CAD build for the part. Positions are in the model's coordinates, mm. A direction names the side the tool comes from. Coordinates: 2 decimals unless noted, no trailing zeros. Loops run counter-clockwise (first coordinate to the right, second up) from the corner with the lowest first, then second, coordinate; pieces in that order, holes last.
1) Pin check, flat tips, straight feed: pin 1 Ø2.5 at (x, z) = (22, 9) entering from +Y; pin 2 Ø10 at (x, y) = (-1.5, -20) entering from +Z; pin 3 Ø2.5 at (x, z) = (21.5, 9) entering from -Y; pin 4 Ø2.5 at (x, y) = (18, 45) entering from -Z. Stop position of each tip, or through.
2) Saw through at C-C, the plane z = 4.5. Write the cut outline in (x, y), and give its area (3 significant figures).
3) Which spindle directions (+Z, -Z, +X, -X, +Y, -Y) get a long thin tool onto all of the face, cutting with end or side? Do faces 1 (the flat face through (0, -25, 1)), 2 (the flat face through (-22, -19.15, 9)), 3 (the flat face through (0, 45, 1)), 4 (the flat face through (-20, 10, 9)). Say none if no direction does.
4) Wall check: line 1 along Y through (x, z) = (-18, 1.65); line 2 along X through (y, z) = (18.5, 8); line 3 along Z through (x, y) = (-11.5, 36). Give the ranges that are in metal, low to high.
5) Saw through at D-D, the plane x = -17.5. Write the cut outline in (y, z), and give its area (3 significant figures).
6) Saw through at B-B, the plane y = 18.5. Write the cut outline in (x, z), and give its area (3 significant figures).
7) Saw through at A-A, the plane x = 18. Write the cut outline in (y, z).
```python
from build123d import *

# Parameters (mm, degrees)
SKETCH1_W           = 40
SKETCH1_H           = 58.3
SKETCH1_R           = 1.55
SKETCH1_W_2         = 3
BOSS_EXTRUDE2_DEPTH = 2.5
SKETCH1_4_W         = 3
SKETCH1_4_H         = 58.3
BOSS_EXTRUDE3_DEPTH = 16
FILLET1_R           = 2
FILLET2_R           = 3


with BuildPart() as part:
    # Sketch1 → Boss-Extrude2 (new body)
    # profile 1 of 5: a face of its own
    with BuildSketch(Plane.XY):
        with Locations((0, 10)):
            Rectangle(SKETCH1_W, SKETCH1_H)
    # profile 2 of 5: a face of its own
    with BuildSketch(Plane.XY):
        Polygon((-23, 39.15), (-20, 39.15), (20, 39.15), (23, 39.15), (23, 50), (13, 50), (13, 45), (-13, 45), (-13, 50), (-23, 50), align=None)
        with Locations((-18, 45)):
            Circle(SKETCH1_R, mode=Mode.SUBTRACT)
        with Locations((18, 45)):
            Circle(SKETCH1_R, mode=Mode.SUBTRACT)
    # profile 3 of 5: a face of its own
    with BuildSketch(Plane.XY):
        with Locations((21.5, 10)):
            Rectangle(SKETCH1_W_2, SKETCH1_H)
    # profile 4 of 5: a face of its own
    with BuildSketch(Plane.XY):
        Polygon((20, -19.15), (-20, -19.15), (-23, -19.15), (-23, -30), (-13, -30), (-13, -25), (13, -25), (13, -30), (23, -30), (23, -19.15), align=None)
        with Locations((-18, -25)):
            Circle(SKETCH1_R, mode=Mode.SUBTRACT)
        with Locations((18, -25)):
            Circle(SKETCH1_R, mode=Mode.SUBTRACT)
    # profile 5 of 5: a face of its own
    with BuildSketch(Plane.XY):
        with Locations((-21.5, 10)):
            Rectangle(SKETCH1_W_2, SKETCH1_H)
    extrude(amount=BOSS_EXTRUDE2_DEPTH)

    # Sketch1_4 → Boss-Extrude3 (add)
    with BuildSketch(Plane.XY):
        with Locations((-21.5, 10)):
            Rectangle(SKETCH1_4_W, SKETCH1_4_H)
        with Locations((21.5, 10)):
            Rectangle(SKETCH1_4_W, SKETCH1_4_H)
    extrude(amount=BOSS_EXTRUDE3_DEPTH)

    # Fillet1
    fillet1_edges = [part.edges().sort_by_distance(p)[0] for p in [
        (13, -30, 1.25),
        (13, -25, 1.25),
        (-13, -25, 1.25),
        (-13, -30, 1.25),
        (-23, -30, 1.25),
        (-23, 50, 1.25),
        (-13, 50, 1.25),
        (-13, 45, 1.25),
        (13, 45, 1.25),
        (13, 50, 1.25),
        (23, 50, 1.25),
        (23, -30, 1.25),
    ]]
    fillet(fillet1_edges, radius=FILLET1_R)

    # Fillet2
    fillet2_edges = [part.edges().sort_by_distance(p)[0] for p in [
        (21.5, 39.15, 2.5),
        (21.5, -19.15, 2.5),
        (-21.5, 39.15, 2.5),
        (-21.5, -19.15, 2.5),
        (-21.5, -19.15, 16),
        (-21.5, 39.15, 16),
        (21.5, 39.15, 16),
        (21.5, -19.15, 16),
    ]]
    fillet(fillet2_edges, radius=FILLET2_R)


solid = part.part
```
Data:
1. pin 1: stops at y = 39.15
1. pin 2: stops at z = 2.5
1. pin 3: stops at y = -19.15
1. pin 4: passes through
2. outline: (-23, -19.32) - (-20, -19.32) - (-20, 39.32) - (-23, 39.32) - close; (20, -19.32) - (23, -19.32) - (23, 39.32) - (20, 39.32) - close
2. area: 352 mm2
3. face 1: +Z, -Z, -Y
3. face 2: +Z, +X, -X, -Y
3. face 3: +Z, -Z, +Y
3. face 4: +Z, +Y, -Y
4. line 1: y = -30 to -26.55, -23.45 to 43.45, 46.55 to 50
4. line 2: x = -23 to -20, 20 to 23
4. line 3: z = 0 to 2.5
5. outline: (-30, 0) - (-26.47, 0) - (-26.47, 2.5) - (-30, 2.5) - close; (-23.53, 0) - (43.53, 0) - (43.53, 2.5) - (-23.53, 2.5) - close; (46.47, 0) - (50, 0) - (50, 2.5) - (46.47, 2.5) - close
5. area: 185 mm2
6. outline: (-23, 0) - (23, 0) - (23, 16) - (20, 16) - (20, 2.5) - (-20, 2.5) - (-20, 16) - (-23, 16) - close
6. area: 196 mm2
7. outline: (-30, 0) - (-26.55, 0) - (-26.55, 2.5) - (-30, 2.5) - close; (-23.45, 0) - (43.45, 0) - (43.45, 2.5) - (-23.45, 2.5) - close; (46.55, 0) - (50, 0) - (50, 2.5) - (46.55, 2.5) - close
